```python
from build123d import *

# Parameters (mm, degrees)
SKETCH1_R           = 1.5
SKETCH1_R_2         = 0.75
BOSS_EXTRUDE1_DEPTH = 4
SKETCH2_R           = 1.25
CUT_EXTRUDE1_DEPTH  = 4
SKETCH3_R           = 1.5
CUT_EXTRUDE2_DEPTH  = 10
SKETCH4_R           = 1.5
SKETCH4_R_2         = 0.75
BOSS_EXTRUDE2_DEPTH = 1
SKETCH5_R           = 2.1
CUT_EXTRUDE3_DEPTH  = 10


with BuildPart() as part:
    # Sketch1 → Boss-Extrude1 (new body)
    with BuildSketch(Plane.XY):
        with BuildLine():
            Line((-81.517614561, 36.788472858), (-36.517614561, 36.788472858))
            ThreePointArc((-36.517614561, 36.788472858), (-31.517614561, 31.788472858), (-36.517614561, 26.788472858))
            Line((-36.517614561, 26.788472858), (-81.517614561, 26.788472858))
            ThreePointArc((-81.517614561, 26.788472858), (-86.517614561, 31.788472858), (-81.517614561, 36.788472858))
        make_face()
        with Locations((-81.517614561, 31.788472858)):
            Circle(SKETCH1_R, mode=Mode.SUBTRACT)
        with Locations((-36.517614561, 31.788472858)):
            Circle(SKETCH1_R_2, mode=Mode.SUBTRACT)
    extrude(amount=BOSS_EXTRUDE1_DEPTH)

    # Sketch2 → Cut-Extrude1 (cut)
    with BuildSketch(Plane.XY.offset(4)):
        with Locations((-71.517614561, 31.788472858)):
            Circle(SKETCH2_R)
    extrude(amount=-CUT_EXTRUDE1_DEPTH, mode=Mode.SUBTRACT)

    # Sketch3 → Cut-Extrude2 (cut)
    with BuildSketch(Plane.XY.offset(4)):
        with Locations((-71.517614561, 31.788472858)):
            Circle(SKETCH3_R)
    extrude(amount=-CUT_EXTRUDE2_DEPTH, mode=Mode.SUBTRACT)

    # Sketch4 → Boss-Extrude2 (add)
    with BuildSketch(Plane.XY.offset(4)):
        with BuildLine():
            Line((-81.517614561, 36.788472858), (-36.517614561, 36.788472858))
            ThreePointArc((-36.517614561, 36.788472858), (-31.517614561, 31.788472858), (-36.517614561, 26.788472858))
            Line((-36.517614561, 26.788472858), (-81.517614561, 26.788472858))
            ThreePointArc((-81.517614561, 26.788472858), (-86.517614561, 31.788472858), (-81.517614561, 36.788472858))
        make_face()
        with Locations((-81.517614561, 31.788472858)):
            Circle(SKETCH4_R, mode=Mode.SUBTRACT)
        with Locations((-71.517614561, 31.788472858)):
            Circle(SKETCH4_R, mode=Mode.SUBTRACT)
        with Locations((-36.517614561, 31.788472858)):
            Circle(SKETCH4_R_2, mode=Mode.SUBTRACT)
    extrude(amount=BOSS_EXTRUDE2_DEPTH)

    # Sketch5 → Cut-Extrude3 (cut)
    with BuildSketch(Plane.XY.offset(5)):
        with Locations((-81.517614561, 31.788472858)):
            Circle(SKETCH5_R)
    extrude(amount=-CUT_EXTRUDE3_DEPTH, mode=Mode.SUBTRACT)


solid = part.part
```
Input: part model. Units: mm. Frame: model coordinates. Give positions to 0.01 mm unless a question says otherwise; leave off trailing zeros. Order: outer loops, then holes, each group sorted by start corner. A loop starts at its lowest first (then second) coordinate and runs counter-clockwise, first axis right, second up. Notation, with made-up numbers: M 39.5,-18 L 81.5,-18 A28 cw 81.5,0 Z; hole C -35.5,32 d2. An arc over 180 degrees is marked long. Return JSON: item names as keys, results as strings.
Item 1: Cut plane A-A (x = -81). Return loops of the section in (y, z).
Solutions:
{"outline": "M 26.79,0 L 29.75,0 L 29.75,5 L 26.79,5 Z; M 33.82,0 L 36.79,0 L 36.79,5 L 33.82,5 Z"}
Item 2: Pull-direction query (X, two-part tool) for faces 1 (the flat face through (-59, 26.788, 2)), 2 (the cylindrical face through (-35.825, 31.501, 2.465)), 3 (the cylindrical face through (-86.516, 31.679, 2.465)), 4 (the cylindrical face through (-79.58, 30.98, 2.54)); classes: +X half, -X half, draft (parallel to the pull), parting line (faces both ways), or undercut.
Solutions:
{"face 1": "draft", "face 2": "undercut", "face 3": "-X half", "face 4": "undercut"}
Item 3: Ray query, probe 1 along X at (y, z) = (30.5, 2.9); probe 2 along X at (y, z) = (31, 4); probe 3 along X at (y, z) = (32.25, 4.35). Return the intervals inside material, ascending.
Solutions:
{"probe 1": "-86.35 to -83.18, -79.86 to -72.29, -70.75 to -31.69", "probe 2": "-86.46 to -83.46, -79.57 to -72.79, -70.24 to -31.58", "probe 3": "-86.5 to -83.57, -79.47 to -72.94, -70.09 to -37.11, -35.93 to -31.54"}
Item 4: First-contact query: P1, Ø1.4, axis at x = -36.52, y = 31.79, coming from the -Z side. Flat tip, straight axial feed; report the tip coordinate or a pass-through.
Solutions:
{"P1": "through"}
Item 5: Cut plane C-C (x = -72.5). Return loops of the section in (y, z).
Solutions:
{"outline": "M 26.79,0 L 30.65,0 L 30.65,5 L 26.79,5 Z; M 32.92,0 L 36.79,0 L 36.79,5 L 32.92,5 Z"}
Item 6: Cut plane B-B (z = 1.85). Return loops of the section in (x, y), then the cut area to 3 significant figures.
Solutions:
{"outline": "M -81.52,26.79 L -36.52,26.79 A5 ccw -36.52,36.79 L -81.52,36.79 A5 ccw Z; hole C -81.52,31.79 d4.2; hole C -71.52,31.79 d3; hole C -36.52,31.79 d1.5", "area": "506 mm^2"}
